Read the model definition and answer for the solid it produces. Units are mm, in the model's axes. A direction names the side the tool comes from. Round coordinates to 2 decimals unless told otherwise and drop trailing zeros. Order: outer loops, then holes, each group sorted by start corner. A loop starts at its lowest first (then second) coordinate and runs counter-clockwise, first axis right, second up. Notation, with made-up numbers: (51.5, -21.5) - (102.5, -21.5) arc R23 ccw to (102.5, 15.5) - close; hole circle Ø9 at (51, -39.5). An arc over 180 degrees is marked (long way). Put each result on its own line as item: value. Start each with the question number.
Q1. Section D-D on x = 11 is taken. Give the vertices of the cut face in (y, z).
Q2. Find the intervals of material crossed by line 1 along Z through (x, y) = (27, -10.25); line 2 along X through (y, z) = (-4.75, 27.5); line 3 along Z through (x, y) = (-28.5, -5.5), in increasing order. Write a range as from..to.
Q3. Section C-C on y = -4 is taken. Give the vertices of the cut face in (x, z).
Q4. Each of these flat-tipped pins is pushed along its axis until it touches: pin 1 Ø12 at (y, z) = (-15.5, -28) entering from +X; pin 2 Ø4 at (x, y) = (16, -21) entering from +Z; pin 3 Ø8 at (y, z) = (-20.5, -12) entering from +X; pin 4 Ø5 at (x, y) = (-14.5, -21) entering from -Z. Where does it stop, or does it pass through?
Q5. Which of the six approach directions +Z, -Z, +X, -X, +Y, -Y give full straight-line access (tool end or side, diameter ignored) to faces 1 (the face through (1, 0, -1)), 2 (the face through (-18.356, -12.522, -27.966))?
Q6. For a pull along Z with two mould halves and no side action, classify faces 3 (the face through (1, -25.4, -1)), 4 (the face through (-33.741, -12.522, 31.314)) as pulls with the +Z half, pulls with the -Z half, needs draft (parallel to the pull), parting line crosses it, or undercut.
Q7. Section A-A on z = -31 is taken. Give the vertices of the cut face in (x, y).
Q8. Section B-B on x = 33.5 is taken. Give the vertices of the cut face in (y, z), then the cut area to 3 significant figures.
from build123d import *

# Parameters (mm, degrees)
F1_DEPTH = 25.4


with BuildPart() as f1:
    # F0 (on Front) → F1 (new body)
    with BuildSketch(Plane.XZ):
        with BuildLine():
            ThreePointArc((-18.735469, 22.730416), (-18.328265, 24.226462), (-18.1911, 25.770856))
            ThreePointArc((-18.1911, 25.770856), (-33.93, 31.074343), (-24.610585, 17.327035))
            ThreePointArc((-24.610585, 17.327035), (-21.02208, 19.320948), (-18.735469, 22.730416))
        make_face()
        with BuildLine():
            ThreePointArc((-18.735469, 22.730416), (-21.02208, 19.320948), (-24.610585, 17.327035))
            ThreePointArc((-24.610585, 17.327035), (-17.469276, -1.99445), (-25.278004, -21.055977))
            ThreePointArc((-25.278004, -21.055977), (-21.412607, -22.868816), (-18.862593, -26.293012))
            ThreePointArc((-18.862593, -26.293012), (1.619037, -19.980616), (21.777358, -27.259737))
            ThreePointArc((21.777358, -27.259737), (23.928897, -23.542629), (27.588285, -21.294319))
            ThreePointArc((27.588285, -21.294319), (18.742727, -1.927072), (27.78602, 17.348638))
            ThreePointArc((27.78602, 17.348638), (24.00136, 19.582777), (21.777358, 23.373403))
            ThreePointArc((21.777358, 23.373403), (1.633225, 15.977432), (-18.735469, 22.730416))
        make_face()
        with BuildLine():
            ThreePointArc((-18.862593, -26.293012), (-21.412607, -22.868816), (-25.278004, -21.055977))
            ThreePointArc((-25.278004, -21.055977), (-33.717153, -35.229558), (-18.1911, -29.657191))
            ThreePointArc((-18.1911, -29.657191), (-18.360613, -27.941921), (-18.862593, -26.293012))
        make_face()
        with BuildLine():
            ThreePointArc((38.969023, 25.770856), (28.995696, 34.44987), (21.777358, 23.373403))
            ThreePointArc((21.777358, 23.373403), (24.00136, 19.582777), (27.78602, 17.348638))
            ThreePointArc((27.78602, 17.348638), (35.47782, 18.770976), (38.969023, 25.770856))
        make_face()
        with BuildLine():
            ThreePointArc((27.588285, -21.294319), (23.928897, -23.542629), (21.777358, -27.259737))
            ThreePointArc((21.777358, -27.259737), (28.995696, -38.336204), (38.969023, -29.657191))
            ThreePointArc((38.969023, -29.657191), (35.394998, -22.595696), (27.588285, -21.294319))
        make_face()
    extrude(amount=F1_DEPTH)


solid = f1.part
Findings:
1. outline: (-25.4, -21.54) - (0, -21.54) - (0, 17.51) - (-25.4, 17.51) - close
2. line 1: -37.81..-20.77, 16.66..33.93
2. line 2: -35.54..-18.36, 21.62..38.8
2. line 3: -38.28..-21.03, 17.15..34.4
3. outline: (-25.28, -21.06) arc R8.76 ccw (long way) to (-18.19, -29.66) arc R8.76 ccw to (-18.86, -26.29) arc R33.79 cw to (21.78, -27.26) arc R8.76 ccw (long way) to (27.59, -21.29) arc R25.34 cw to (27.79, 17.35) arc R8.76 ccw (long way) to (21.78, 23.37) arc R32.54 cw to (-18.74, 22.73) arc R8.76 ccw to (-18.19, 25.77) arc R8.76 ccw (long way) to (-24.61, 17.33) arc R28.38 cw to start
4. pin 1: x = 38.97
4. pin 2: z = 20.7
4. pin 3: x = 22.92
4. pin 4: z = -25.05
5. face 1: +Z, -Z, +X, -X, +Y
5. face 2: +Y, -Y
6. face 3: needs draft
6. face 4: undercut
7. outline: (-35.61, -25.4) - (-18.29, -25.4) - (-18.29, 0) - (-35.61, 0) - close; (21.55, -25.4) - (38.87, -25.4) - (38.87, 0) - (21.55, 0) - close
8. outline: (-25.4, -37.78) - (0, -37.78) - (0, -21.54) - (-25.4, -21.54) - close; (-25.4, 17.65) - (0, 17.65) - (0, 33.89) - (-25.4, 33.89) - close
8. area: 825 mm2
